Check sheet for the drawn part. Datum: minimum x, y, z corner. Units: mm. Coordinates: 2 decimals unless noted, no trailing zeros. Loops run counter-clockwise (first coordinate to the right, second up) from the corner with the lowest first, then second, coordinate; pieces in that order, holes last.
Q1. Sectioned sample at A-A (x = 5). Enter the section's corners in (y, z), then the cut area to 3 significant figures.
Q2. Sectioned sample at C-C (z = 0.35). Enter the section's corners in (x, y), then the cut area to 3 significant figures.
Q3. Material ranges on probe 1 along Y at (x, z) = (5, 0.4); probe 2 along Y at (x, z) = (3.75, 0.5); probe 3 along X at (y, z) = (27.75, 0.55), recorded low to high.
Q4. Sectioned sample at B-B (y = 3.5). Enter the section's corners in (x, z).
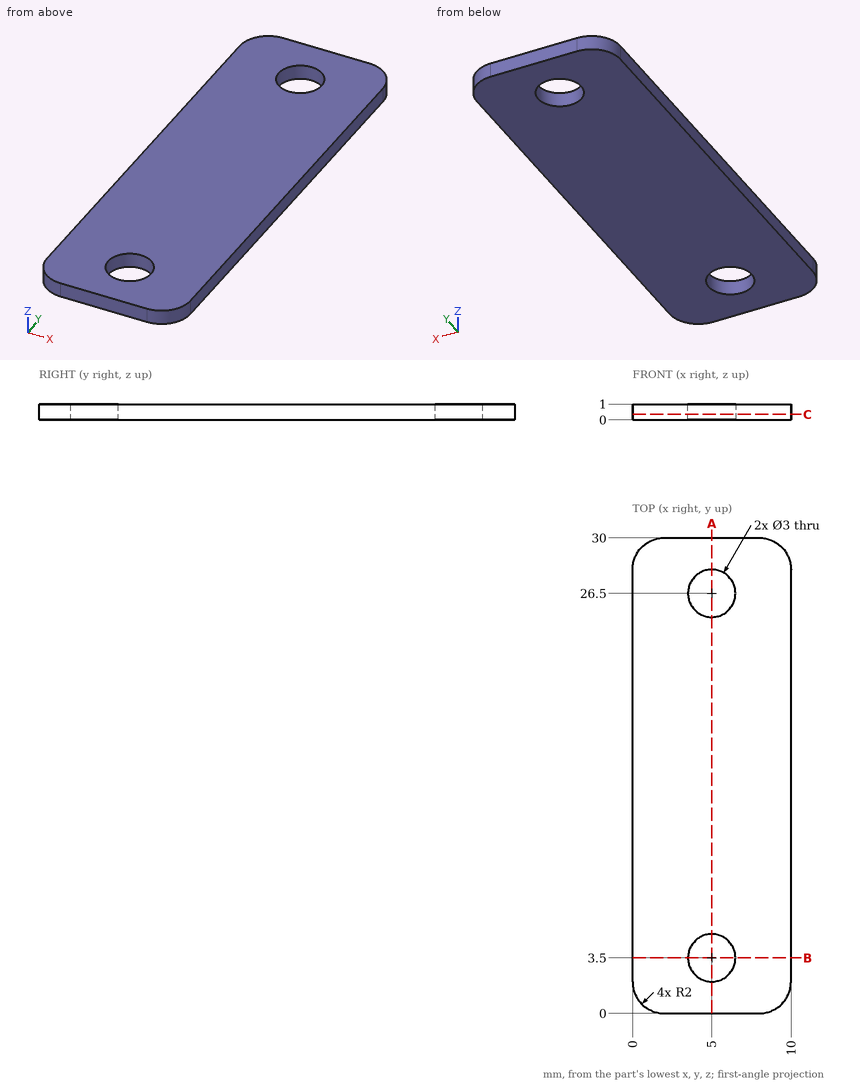
Geometry check:
1. outline: (0, 0) - (2, 0) - (2, 1) - (0, 1) - close; (5, 0) - (25, 0) - (25, 1) - (5, 1) - close; (28, 0) - (30, 0) - (30, 1) - (28, 1) - close
1. area: 24.0 mm2
2. outline: (0, 2) arc R2 ccw to (2, 0) - (8, 0) arc R2 ccw to (10, 2) - (10, 28) arc R2 ccw to (8, 30) - (2, 30) arc R2 ccw to (0, 28) - close; hole circle Ø3 at (5, 3.5); hole circle Ø3 at (5, 26.5)
2. area: 282 mm2
3. probe 1: y = 0 to 2, 5 to 25, 28 to 30
3. probe 2: y = 0 to 2.67, 4.33 to 25.67, 27.33 to 30
3. probe 3: x = 0 to 4.17, 5.83 to 10
4. outline: (0, 0) - (3.5, 0) - (3.5, 1) - (0, 1) - close; (6.5, 0) - (10, 0) - (10, 1) - (6.5, 1) - close
